```python
from build123d import *

# Parameters (mm, degrees)
FILLET1_R   = 0.1
HEX_2_DEPTH = 1.1


with BuildPart() as part:
    # BodySke → BaseBody (revolve)
    with BuildSketch(Plane.XY):
        Polygon((0, 0), (0, 2.675), (0.685, 2.675), (1.86, 1.5), (5.7195, 1.5), (6, 1.2195), (6, 0), align=None)
    revolve(axis=Axis((0, 0, 0), (1, 0, 0)))

    # Fillet1
    fillet1_edges = [part.edges().sort_by_distance(p)[0] for p in [
        (1.86, -1.5, 0),
    ]]
    fillet(fillet1_edges, radius=FILLET1_R)

    # Sketch2 → PreBroach (revolve, cut)
    with BuildSketch(Plane.XY):
        Polygon((0, 1), (1.1, 1), (1.677350269, 0), (0, 0), align=None)
    revolve(axis=Axis((0, 0, 0), (1, 0, 0)), mode=Mode.SUBTRACT)

    # Sketch3 → Hex 2 (cut)
    with BuildSketch(Plane.ZY):
        Polygon((-1, -0.577350269), (-1, 0.577350269), (0, 1.154700538), (1, 0.577350269), (1, -0.577350269), (0, -1.154700538), align=None)
    extrude(amount=-HEX_2_DEPTH, mode=Mode.SUBTRACT)


solid = part.part
```
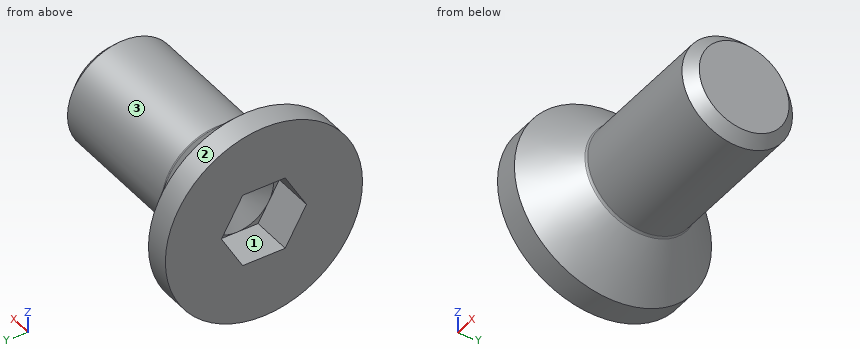
Could you check a few things on this model? Use its own coordinates, in mm. Face numbers are marked on the shaded views. A direction names the side the tool comes from. Give positions to 0.01 mm unless a question says otherwise; leave off trailing zeros. Loops run counter-clockwise (first coordinate to the right, second up) from the corner with the lowest first, then second, coordinate; pieces in that order, holes last. Notation, with made-up numbers: (80.25, -28) - (132.25, -28) arc R27 ccw to (132.25, 11) - close; hole circle Ø1 at (25, 78). An arc over 180 degrees is marked (long way). Answer in a Markdown table with one row per item. Add a question column.
Q1. If we section it at B-B (x = 4.25): List the corners of the cut face in (y, z) for me.
Q2. Please list where these lines run through material, in increasing order: L1, parallel to Y at x = 0.4, z = 0.2; L2, parallel to Z at x = 0.9, y = -1; L3, parallel to Y at x = 0.6, z = 0.8. Write a range as from..to.
Q3. Which directions (+Z, -Z, +X, -X, +Y, -Y) give clear straight access to the entire face, cutting with the end or side of a thin tool? Please do the marked faces 1, 2 and 3.
Q4. For pin 1 (1 mm diameter, centred on x = 2.5, z = -1, fed in from +Y); pin 2 (1.5 mm diameter, centred on y = 2, z = 0, fed in from +X); pin 3 (3 mm diameter, centred on x = 3.5, y = -0.5, fed in from +Z), each with a flat end and sliding along its axis, tell me the tip position at first contact or that it passes through.
Q5. If we section it at A-A (x = 0.8): List the corners of the cut face in (y, z) for me, plus the area to 3 significant figures.
The answers:
| question | item | result |
|---|---|---|
| 1 | outline | circle Ø3 at (0, 0) |
| 2 | L1 | y = -2.67..-1.04, 1.04..2.67 |
| 2 | L2 | z = -2.25..-0.27, 0.27..2.25 |
| 2 | L3 | y = -2.55..-0.69, 0.69..2.55 |
| 3 | face 1 | -X |
| 3 | face 2 | +X, -X |
| 3 | face 3 | +X |
| 4 | pin 1 | stops at y = 1.41 |
| 4 | pin 2 | stops at x = 5.97 |
| 4 | pin 3 | stops at z = 1.5 |
| 5 | outline | circle Ø5.12 at (0, 0); hole (-1.15, 0) - (-0.58, -1) - (0.58, -1) - (1.15, 0) - (0.58, 1) - (-0.58, 1) - close |
| 5 | area | 17.1 mm^2 |
